```python
from build123d import *

# Parameters (mm, degrees)
SKETCH1_R           = 55
BOSS_EXTRUDE1_DEPTH = 100
FILLET1_R           = 10
SKETCH3_R           = 50
CUT_EXTRUDE1_DEPTH  = 90


with BuildPart() as part:
    # Sketch1 → Boss-Extrude1 (new body)
    with BuildSketch(Plane(origin=(0, 0, 0), x_dir=(1, 0, 0), z_dir=(0, 1, 0))):
        with Locations(Location((0, 0, 0), (0, 0, 270))):
            Circle(SKETCH1_R)
    extrude(amount=BOSS_EXTRUDE1_DEPTH)

    # Fillet1
    fillet1_edges = [part.edges().sort_by_distance(p)[0] for p in [
        (0, 0, -55),
        (0, 100, -55),
    ]]
    fillet(fillet1_edges, radius=FILLET1_R)

    # Sketch3 → Cut-Extrude1 (cut)
    with BuildSketch(Plane(origin=(0, 100, 0), x_dir=(1, 0, 0), z_dir=(0, 1, 0))):
        with Locations(Location((0, 0, 0), (0, 0, 270))):
            Circle(SKETCH3_R)
    extrude(amount=-CUT_EXTRUDE1_DEPTH, mode=Mode.SUBTRACT)


solid = part.part
```
Could you check a few things on this model? Use its own coordinates, in mm. Coordinates: 2 decimals unless noted, no trailing zeros. Loops run counter-clockwise (first coordinate to the right, second up) from the corner with the lowest first, then second, coordinate; pieces in that order, holes last.
1) Imagine slicing it at C-C (y = 60.5). List the corners of the cut face in (x, z) for me.
Reported:
outline: circle Ø110 at (0, 0); hole circle Ø100 at (0, 0)
2) Thinking about a two-plate mould opening in Z: for faces 1 (the face through (-48.794, 49.44, 25.379)), 2 (the face through (1, 0, -1)), 3 (the face through (15.02, 54.95, 47.69)), which applies, released by +Z, released by -Z, zero draft, split by the parting line, or undercut?
Reported:
face 1: split by the parting line
face 2: zero draft
face 3: undercut
3) Imagine slicing it at A-A (x = 0). List the corners of the cut face in (y, z) for me, and give its area (3 significant figures).
Reported:
outline: (0, -45) arc R10 ccw to (10, -55) - (90, -55) arc R10 ccw to (98.66, -50) - (10, -50) - (10, 50) - (98.66, 50) arc R10 ccw to (90, 55) - (10, 55) arc R10 ccw to (0, 45) - close
area: 1,920 mm2
4) Will these pins go through, and if not, where does the flat tip stop? pin 1 Ø3 at (x, z) = (20.5, 9) entering from +Y; pin 2 Ø1.5 at (x, y) = (41.5, 81) entering from +Z; pin 3 Ø3 at (y, z) = (46.5, 16) entering from +X; pin 4 Ø6 at (x, z) = (38.5, -8.5) entering from -Y.
Reported:
pin 1: stops at y = 10
pin 2: stops at z = 36.94
pin 3: stops at x = 53.05
pin 4: stops at y = 0
5) Please list where these lines run through material, in increasing order: line 1 along Z through (x, y) = (-1.5, 75); line 2 along X through (y, z) = (49, 0); line 3 along Y through (x, z) = (6, -32).
Reported:
line 1: z = -54.98 to -49.98, 49.98 to 54.98
line 2: x = -55 to -50, 50 to 55
line 3: y = 0 to 10
6) Imagine slicing it at D-D (y = 92.5). List the corners of the cut face in (x, z) for me.
Reported:
outline: circle Ø109.36 at (0, 0); hole circle Ø100 at (0, 0)
7) Imagine slicing it at B-B (z = 0). List the corners of the cut face in (x, y) for me.
Reported:
outline: (-55, 10) arc R10 ccw to (-45, 0) - (45, 0) arc R10 ccw to (55, 10) - (55, 90) arc R10 ccw to (50, 98.66) - (50, 10) - (-50, 10) - (-50, 98.66) arc R10 ccw to (-55, 90) - close
